Check sheet for the modelled part. Datum: model origin and axes. Units: mm. A direction names the side the tool comes from. Give positions to 0.01 mm unless a question says otherwise; leave off trailing zeros. Write each loop counter-clockwise with the first axis right and the second up, starting at its lowest first coordinate (ties: lowest second). Pieces come first, ordered by that corner, then holes. Notation, with made-up numbers: M -5.75,69.5 L 19.25,69.5 A18 ccw 19.25,84.5 Z; hole C 76.5,74 d9. An arc over 180 degrees is marked long. Write item = value, one per line. Start each with the question number.
1) Cross-section at D-D, the plane z = 16.5. Record the cut outline in (x, y), plus the area to 3 significant figures.
2) Mould release check, pull along X, two halves, no side actions. Record for faces 4 (the flat face through (2.25, 0, -3)), 5 (the flat face through (78.01, 0.02, 2.31)): released by +X, released by -X, zero draft, split by the parting line, or undercut.
3) Cross-section at B-B, the plane z = 7. Record the cut outline in (x, y).
4) Scan lines: line 1 along X through (y, z) = (0.85, -15.5); line 2 along X through (y, z) = (0.15, 16.5); line 3 along X through (y, z) = (-0.75, -3). Record each from-to range of solid material in increasing order. Write a range as [from, to].
5) Cross-section at A-A, the plane x = 55. Record the cut outline in (y, z), plus the area to 3 significant figures.
6) Access from +Z, -Z, +X, -X, +Y, -Y to the whole of each face (thin tool, end or side, straight path). Record for faces 1 (the flat face through (21, 0, -18.678)), 2 (the flat face through (49.65, 0.02, 12.36)), 3 (the flat face through (10.5, 0, -4)).
7) Cross-section at C-C, the plane y = 0.15. Give the number of separate pieces and of enclosed holes in the cut face, plus the area to 3 significant figures.
8) Go/stop test with flat-tipped pins: pin 1 (1.5 mm diameter, centred on x = 4.5, y = 0.5, fed in from -Z); pin 2 (0.9 mm diameter, centred on y = -0.5, z = -4.5, fed in from -X); pin 3 (1.5 mm diameter, centred on x = 13, y = 0.5, fed in from +Z). Record where each tip stops, or that it passes through.
```python
from build123d import *

# Parameters (mm, degrees)
SKETCH_1_W          = 182
SKETCH_1_H          = 40
EXTRUDE_1_DEPTH     = 1.5
SKETCH_2_R          = 1.5
CUT_EXTRUDE_1_DEPTH = 94.220169491
SKETCH_3_R          = 1.6
CUT_EXTRUDE_2_DEPTH = 94.220169491
CUT_EXTRUDE_3_DEPTH = 94.220169491
CUT_EXTRUDE_4_DEPTH = 93.146676554


with BuildPart() as part:
    # 草图1 → 凸台-拉伸1 (new, symmetric)
    with BuildSketch(Plane(origin=(0, 0, 0), x_dir=(1, 0, 0), z_dir=(0, 1, 0))):
        Rectangle(SKETCH_1_W, SKETCH_1_H)
    extrude(amount=EXTRUDE_1_DEPTH, both=True)

    # 草图2 → 切除-拉伸1 (cut, through all)
    with BuildSketch(Plane(origin=(0, 1.5, 0), x_dir=(1, 0, 0), z_dir=(0, 1, 0))):
        with Locations(Location((-86.4, 15.5, 0), (0, 0, 270))):
            Circle(SKETCH_2_R)
        with Locations(Location((-63.6, -16.5, 0), (0, 0, 270))):
            Circle(SKETCH_2_R)
        with Locations(Location((63.6, -16.5, 0), (0, 0, 90))):
            Circle(SKETCH_2_R)
        with Locations(Location((86.4, 15.5, 0), (0, 0, 90))):
            Circle(SKETCH_2_R)
    extrude(amount=-CUT_EXTRUDE_1_DEPTH, mode=Mode.SUBTRACT)

    # 草图3 → 切除-拉伸2 (cut, through all)
    with BuildSketch(Plane(origin=(0, 1.5, 0), x_dir=(1, 0, 0), z_dir=(0, 1, 0))):
        with Locations(Location((-10, 15, 0), (0, 0, 270))):
            Circle(SKETCH_3_R)
        with Locations(Location((10, 15, 0), (0, 0, 90))):
            Circle(SKETCH_3_R)
        Polygon((5.5, 20), (-5.5, 20), (-5.5, 6), (-2.25, 6), (-2.25, 0), (2.25, 0), (2.25, 6), (5.5, 6), align=None)
    extrude(amount=-CUT_EXTRUDE_2_DEPTH, mode=Mode.SUBTRACT)

    # 草图4 → 切除-拉伸3 (cut, through all)
    with BuildSketch(Plane(origin=(0, 1.5, 0), x_dir=(1, 0, 0), z_dir=(0, 1, 0))):
        Polygon((-79.576847618, 11.955270909), (-62.609658275, -11.858328169), (-22.72187982, 11.583183423), align=None)
        with BuildLine():
            ThreePointArc((-89.250472649, 13.469038238), (-89.505875328, 17.113548403), (-86.377094731, 18.999925049))
            Line((-86.377094731, 18.999925049), (-37.123877911, 18.677587243))
            Line((-37.123877911, 18.677587243), (-5.5, 18.677587243))
            Line((-5.5, 18.677587243), (-5.5, 20))
            Line((-5.5, 20), (-91, 20))
            Line((-91, 20), (-91, -20))
            Line((-91, -20), (-63.6, -20))
            ThreePointArc((-63.6, -20), (-65.203376723, -19.611138551), (-66.450472649, -18.530961762))
            Line((-66.450472649, -18.530961762), (-89.250472649, 13.469038238))
        make_face()
        with BuildLine():
            Line((-37.123877911, -5), (-61.826659834, -19.517493108))
            ThreePointArc((-61.826659834, -19.517493108), (-62.68109464, -19.877219705), (-63.6, -20))
            Line((-63.6, -20), (63.600000006, -20))
            ThreePointArc((63.600000006, -20), (62.681094642, -19.877219706), (61.826659834, -19.517493108))
            Line((61.826659834, -19.517493108), (37.123877911, -5))
            Line((37.123877911, -5), (-37.123877911, -5))
        make_face()
        with BuildLine():
            Line((5.5, 20), (5.5, 18.677587243))
            Line((5.5, 18.677587243), (37.123877911, 18.677587243))
            Line((37.123877911, 18.677587243), (86.377094731, 18.999925049))
            ThreePointArc((86.377094731, 18.999925049), (89.505875328, 17.113548403), (89.250472649, 13.469038238))
            Line((89.250472649, 13.469038238), (66.450472649, -18.530961762))
            ThreePointArc((66.450472649, -18.530961762), (65.203376726, -19.61113855), (63.600000006, -20))
            Line((63.600000006, -20), (91, -20))
            Line((91, -20), (91, 20))
            Line((91, 20), (5.5, 20))
        make_face()
        Polygon((79.576847618, 11.955270909), (22.72187982, 11.583183423), (62.609658275, -11.858328169), align=None)
    extrude(amount=-CUT_EXTRUDE_3_DEPTH, mode=Mode.SUBTRACT)

    # 草图5 → 切除-拉伸4 (cut, through all)
    with BuildSketch(Plane(origin=(0, 1.5, 0), x_dir=(1, 0, 0), z_dir=(0, 1, 0))):
        Polygon((-17.797622354, 8.677587243), (-32.563294615, 0), (-10.5, 0), (-10.5, 8.677587243), align=None)
        Polygon((17.797622354, 8.677587243), (10.5, 8.677587243), (10.5, 0), (32.563294615, 0), align=None)
    extrude(amount=-CUT_EXTRUDE_4_DEPTH, mode=Mode.SUBTRACT)


solid = part.part
```
Reply:
q1.outline = M -67.9,-1.5 L -65.1,-1.5 L -65.1,1.5 L -67.9,1.5 Z; M -62.1,-1.5 L -56.69,-1.5 L -56.69,1.5 L -62.1,1.5 Z; M 56.69,-1.5 L 62.1,-1.5 L 62.1,1.5 L 56.69,1.5 Z; M 65.1,-1.5 L 67.9,-1.5 L 67.9,1.5 L 65.1,1.5 Z
q1.area = 49.2 mm2
q2.face_4 = undercut
q2.face_5 = released by +X
q3.outline = M -74.67,-1.5 L -66.07,-1.5 L -66.07,1.5 L -74.67,1.5 Z; M -54.34,-1.5 L -40.53,-1.5 L -40.53,1.5 L -54.34,1.5 Z; M 40.53,-1.5 L 54.34,-1.5 L 54.34,1.5 L 40.53,1.5 Z; M 66.07,-1.5 L 74.67,-1.5 L 74.67,1.5 L 66.07,1.5 Z
q4.line_1 = [-89.9, -87.9], [-84.9, -11.52], [-8.48, -5.5], [5.5, 8.48], [11.52, 84.9], [87.9, 89.9]
q4.line_2 = [-67.9, -65.1], [-62.1, -56.69], [56.69, 62.1], [65.1, 67.9]
q4.line_3 = [-81.79, -73.2], [-37.33, -27.46], [-10.5, -2.25], [2.25, 10.5], [27.46, 37.33], [73.2, 81.79]
q5.outline = M -1.5,-18.79 L 1.5,-18.79 L 1.5,-11.79 L -1.5,-11.79 Z; M -1.5,7.39 L 1.5,7.39 L 1.5,15.51 L -1.5,15.51 Z
q5.area = 45.4 mm2
q6.face_1 = -Z, +Y, -Y
q6.face_2 = +Z, +Y, -Y
q6.face_3 = +Y, -Y
q7.separate_pieces = 1
q7.enclosed_holes = 10
q7.area = 2,810 mm2
q8.pin_1 = -6
q8.pin_2 = -83.18
q8.pin_3 = 5
